```python
from build123d import *

# Parameters (mm, degrees)
F0_W     = 82.5
F0_H     = 20
F1_DEPTH = 8
F2_D     = 10.2
F3_D     = 6.8
F4_R     = 9.99999


# Not quite as in the source:
# - a fillet or chamfer is up to 0.001 mm smaller than in the source, because OpenCascade refuses the exact size


with BuildPart() as f1:
    # F0 (on Top) → F1 (new body)
    with BuildSketch(Plane.XY):
        Rectangle(F0_W, F0_H)
    extrude(amount=-F1_DEPTH)

    # F2 (through all)
    with Locations(Plane.XY):
        with Locations((-31.25, 0)):
            Hole(F2_D / 2)

    # F3 (through all)
    with Locations(Plane.XY):
        with Locations((31.25, 0)):
            Hole(F3_D / 2)

    # F4 (radius 10 in the source; OpenCascade refuses exactly that, so slightly less here)
    f4_edges = [f1.edges().sort_by_distance(p)[0] for p in [
        (41.25, 10, -4),
        (41.25, -10, -4),
        (-41.25, 10, -4),
        (-41.25, -10, -4),
    ]]
    fillet(f4_edges, radius=F4_R)


solid = f1.part
```
Could you check a few things on this model? Use its own coordinates, in mm. Round coordinates to 2 decimals unless told otherwise and drop trailing zeros. Loops run counter-clockwise (first coordinate to the right, second up) from the corner with the lowest first, then second, coordinate; pieces in that order, holes last.
Q1. I want a section at B-B (y = -4.25). Write out the boundary of the cut face in (x, z).
Q2. Please list where these lines run through material, in increasing order: L1, parallel to Y at x = 31.25, z = -4; L2, parallel to X at y = -3, z = -1.75; L3, parallel to X at y = -6.5, z = -1.5.
Q3. Thinking about a two-plate mould opening in X: for faces 1 (the cylindrical face through (-26.155, 0.224, -4.056)), 2 (the cylindrical face through (-38.4, 6.99, -4.06)), 3 (the flat face through (0, 10, -4)), which applies, pulls with the +X half, pulls with the -X half, needs draft (parallel to the pull), parting line crosses it, or undercut?
Q4. I want a section at A-A (z = -2.25). Give the number of separate pieces and of enclosed holes in the cut face, and give its area (3 significant figures).
Answer below:
1. outline: (-40.3, -8) - (-34.07, -8) - (-34.07, 0) - (-40.3, 0) - close; (-28.43, -8) - (40.3, -8) - (40.3, 0) - (-28.43, 0) - close
2. L1: y = -10 to -3.4, 3.4 to 10
2. L2: x = -40.79 to -35.37, -27.13 to 29.65, 32.85 to 40.79
2. L3: x = -38.85 to 38.85
3. face 1: undercut
3. face 2: pulls with the -X half
3. face 3: needs draft
4. separate pieces: 1
4. enclosed holes: 2
4. area: 1,450 mm2
